Model file for the job. Use its own axes, mm. Face numbers are marked on the shaded views. Coordinates: 2 decimals unless noted, no trailing zeros. Order: outer loops, then holes, each group sorted by start corner. A loop starts at its lowest first (then second) coordinate and runs counter-clockwise, first axis right, second up. Notation, with made-up numbers: (85.25, -29.75) -> (124.25, -29.75) arc R26 cw to (124.25, 9.25) -> close; hole circle Ø1 at (29.5, 71.25). An arc over 180 degrees is marked (long way). Return JSON: item names as keys, results as strings. Group by question number.
1) Probe line 1 (Y direction, x = 7, z = 1.25); line 2 (Y direction, x = 17.5, z = 1.95); line 3 (Y direction, x = 25.1, z = 1.4). List the from-to ranges inside material, lowest first.
2) Flat gauge pins, fed straight in: pin 1 (5 mm diameter, centred on x = 28, y = 75.4, fed in from +Z); pin 2 (1.5 mm diameter, centred on x = 150, z = 1, fed in from +Y); pin 3 (1 mm diameter, centred on y = 67, z = 1.5, fed in from +X). Where does each tip first touch, or does it go through?
3) Cut at D-D (x = 163.1). Write the cut outline in (y, z).
4) Cut at A-A (y = 64.9). Write the cut outline in (x, z).
5) Cut at B-B (y = 75.4). Write the cut outline in (x, z).
6) Cut at C-C (z = 3.7). State how many separate pieces and enclosed holes the cut face has, and give its area (3 significant figures).
7) Pull direction X, two halves, no side cores. Call the marked faces 1 and 2: +X half, -X half, draft (parallel to the pull), parting line (faces both ways), or undercut.
from build123d import *

# Parameters (mm, degrees)
SKETCH1_R            = 2.7
BOSS_EXTRUDE1_DEPTH  = 3
SKETCH3_R            = 2.995
BOSS_EXTRUDE2_DEPTH  = 1.4
LPATTERN1_COUNT      = 2
LPATTERN1_PITCH      = 23
LPATTERN1_COUNT_DIR2 = 11
LPATTERN1_PITCH_DIR2 = 23
FILLET2_R            = 4
SKETCH5_R            = 4.25
SKETCH5_R_2          = 2.25
CUT_EXTRUDE2_DEPTH   = 271.093687449


with BuildPart() as part:
    # Sketch1 → Boss-Extrude1 (new body)
    with BuildSketch(Plane.XY):
        Polygon((0, 0), (257.2, 0), (257.2, 47.4), (70, 47.4), (35, 82.4), (0, 82.4), (0, 47.4), align=None)
        with Locations((232.1, 23.7)):
            Circle(SKETCH1_R, mode=Mode.SUBTRACT)
        with Locations((163.1, 23.7)):
            Circle(SKETCH1_R, mode=Mode.SUBTRACT)
        with Locations((94.1, 23.7)):
            Circle(SKETCH1_R, mode=Mode.SUBTRACT)
        with Locations((25.1, 23.7)):
            Circle(SKETCH1_R, mode=Mode.SUBTRACT)
    extrude(amount=BOSS_EXTRUDE1_DEPTH)

    # Sketch3 → Boss-Extrude2 (add)
    with BuildSketch(Plane.XY.offset(3)):
        with Locations(Location((13.6, 12.2, 0), (0, 0, 180))):
            Circle(SKETCH3_R)
    boss_extrude2 = extrude(amount=BOSS_EXTRUDE2_DEPTH)

    # LPattern1: Boss-Extrude2 2 × 11
    with Locations(*[(j * LPATTERN1_PITCH_DIR2, i * LPATTERN1_PITCH, 0) for i in range(LPATTERN1_COUNT) for j in range(LPATTERN1_COUNT_DIR2) if (i, j) != (0, 0)]):
        add(boss_extrude2)

    # Fillet2
    fillet2_edges = [part.edges().sort_by_distance(p)[0] for p in [
        (0, 82.4, 1.5),
        (35, 82.4, 1.5),
        (70, 47.4, 1.5),
    ]]
    fillet(fillet2_edges, radius=FILLET2_R)

    # Sketch5 → Cut-Extrude2 (cut, through all)
    with BuildSketch(Plane.XY.offset(3)):
        with Locations((17.5, 64.9)):
            Circle(SKETCH5_R)
        with Locations((7, 75.4)):
            Circle(SKETCH5_R_2)
        with Locations((28, 75.4)):
            Circle(SKETCH5_R_2)
        with Locations((28, 54.4)):
            Circle(SKETCH5_R_2)
        with Locations((7, 54.4)):
            Circle(SKETCH5_R_2)
    extrude(amount=-CUT_EXTRUDE2_DEPTH, mode=Mode.SUBTRACT)


solid = part.part
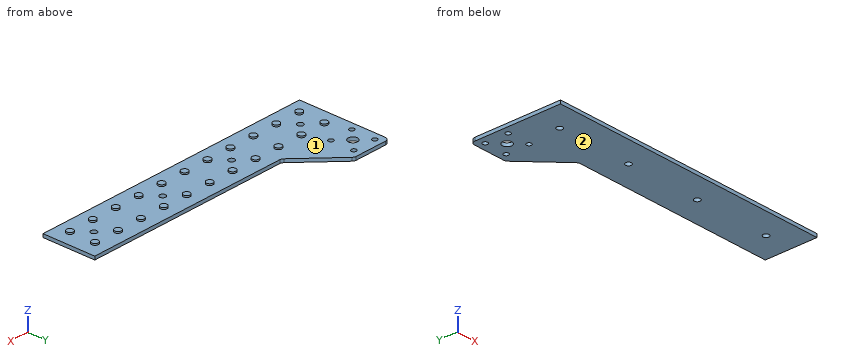
Answers below:
{
 "1": {"line 1": "y = 0 to 52.15, 56.65 to 73.15, 77.65 to 82.4", "line 2": "y = 0 to 60.65, 69.15 to 82.4", "line 3": "y = 0 to 21, 26.4 to 82.4"},
 "2": {"pin 1": "stops at z = 3", "pin 2": "stops at y = 47.4", "pin 3": "stops at x = 50.9"},
 "3": {"outline": "(0, 0) -> (21, 0) -> (21, 3) -> (0, 3) -> close; (26.4, 0) -> (47.4, 0) -> (47.4, 3) -> (26.4, 3) -> close"},
 "4": {"outline": "(0, 0) -> (13.25, 0) -> (13.25, 3) -> (0, 3) -> close; (21.75, 0) -> (52.5, 0) -> (52.5, 3) -> (21.75, 3) -> close"},
 "5": {"outline": "(0, 0) -> (4.75, 0) -> (4.75, 3) -> (0, 3) -> close; (9.25, 0) -> (25.75, 0) -> (25.75, 3) -> (9.25, 3) -> close; (30.25, 0) -> (42, 0) -> (42, 3) -> (30.25, 3) -> close"},
 "6": {"separate pieces": "22", "enclosed holes": "0", "area": "620 mm^2"},
 "7": {"face 1": "undercut", "face 2": "draft"}
}
